The model under review builds one solid part; all positions refer to its coordinate system, in mm. Coordinates: 2 decimals unless noted, no trailing zeros. Write each loop counter-clockwise with the first axis right and the second up, starting at its lowest first coordinate (ties: lowest second). Pieces come first, ordered by that corner, then holes.
```python
from build123d import *

# Parameters (mm, degrees)
F1_DEPTH = 25.4
F2_R     = 5.08


with BuildPart() as f1:
    # F0 (on Top) → F1 (new body)
    with BuildSketch(Plane.XY):
        Polygon((-24.859279, 47.311023), (0, 0), (96.377738, 0), (96.377738, 47.311023), align=None)
    extrude(amount=F1_DEPTH)

    # F2
    f2_edges = [f1.edges().sort_by_distance(p)[0] for p in [
        (-12.42964, 23.655511, 25.4),
        (35.759229, 47.311023, 25.4),
        (96.377738, 23.655511, 25.4),
        (96.377738, 47.311023, 12.7),
    ]]
    fillet(f2_edges, radius=F2_R)


solid = f1.part
```
Item 1: To check wall thickness, follow line 1 along Y through (x, z) = (91.5, 14.75); line 2 along Y through (x, z) = (-14.5, 18.25); line 3 along X through (y, z) = (43, 13.25). State the ranges of each line that lie inside material, in increasing order.
Solved:
line 1: y = 0 to 47.31
line 2: y = 27.6 to 47.31
line 3: x = -22.59 to 96.32
Item 2: Take a section at A-A, the plane z = 19. Write out the cut boundary in (x, y), plus the area to 3 significant figures.
Solved:
outline: (-24.86, 47.31) - (0, 0) - (96.38, 0) - (96.38, 42.23) arc R5.08 ccw to (91.3, 47.31) - close
area: 5,140 mm2
Item 3: For pin 1 (10 mm diameter, centred on y = 31.5, z = 13, fed in from -X); pin 2 (10 mm diameter, centred on y = 8.5, z = 4.5, fed in from -X), all flat-tipped, find the tip position at first contact; note any pin that passes through.
Solved:
pin 1: stops at x = -19.18
pin 2: stops at x = -7.09
